Autodesk Inventor part; units mm, degrees
ref_plane "YZ Plane" through (0, 0, 0) normal (1, 0, 0) x (0, 1, 0)
ref_plane "XZ Plane" through (0, 0, 0) normal (0, 1, 0) x (-1, 0, 0)
ref_plane "XY Plane" through (0, 0, 0) normal (0, 0, 1) x (1, 0, 0)
sketch "スケッチ2" plane through (0, 0, 0) normal (0, 0, 1) x (1, 0, 0)
  line L0 (0, 0) -> (20, 0)
  line L1 (20, 0) -> (20, 80)
  line L2 (20, 80) -> (0, 80)
  line L3 (0, 80) -> (0, 0)
  line L4 (10, 80) -> (10, 0) construction
  circle A0 centre (10, 70) radius 2.75
  circle A1 centre (10, 10) radius 2.75
  dimension "d4" = 20
  dimension "d5" = 80
  dimension "d15" = 10
  dimension "d16" = 10
  dimension "d17" = 5.5
extrude "押し出し2" add sketch "スケッチ2" along normal blind 25
sketch "スケッチ4" plane through (0, 0, 25) normal (0, 0, 1) x (1, 0, 0)
  line L0 (0, 0) -> (20, 0) construction
  line L1 (10, 0) -> (10, 80) construction
  line L2 (20, 80) -> (0, 80) construction
  line L3 (0, 80) -> (0, 0) construction
  line L4 (0, 40) -> (20, 40) construction
  line L5 (20, 0) -> (20, 80) construction
  line L6 (13, 25) -> (7, 25)
  line L7 (7, 25) -> (7, 55)
  line L8 (7, 55) -> (13, 55)
  line L9 (13, 55) -> (13, 25)
  line L10 (13, 25) -> (7, 55) construction
  line L11 (7, 25) -> (13, 55) construction
  point P0 (10, 40)
  dimension "d18" = 6
  dimension "d19" = 30
extrude "押し出し4" add sketch "スケッチ4" along normal blind 2
fillet "フィレット1" radius 1 8 edges at (13, 25, 26) (13, 55, 26) (7, 55, 26) (7, 25, 26) (0, 0, 12.5) (20, 0, 12.5) (20, 80, 12.5) (0, 80, 12.5)
properties part number "モータースペーサ"
Could you check a few things on this model? Use its own coordinates, in mm. A direction names the side the tool comes from. Round coordinates to 2 decimals unless told otherwise and drop trailing zeros. Order: outer loops, then holes, each group sorted by start corner. A loop starts at its lowest first (then second) coordinate and runs counter-clockwise, first axis right, second up. Notation, with made-up numbers: M 47.25,-33 L 64.25,-33 A9 cw 64.25,-29 Z; hole C 62.5,-23.5 d6. An arc over 180 degrees is marked long. One line per item, written item: value.
(1) Which directions (+Z, -Z, +X, -X, +Y, -Y) give clear straight access to the entire face, cutting with the end or side of a thin tool? Please do faces 1 (the flat face through (10, 55, 26)), 2 (the flat face through (7, 40, 26)), 3 (the flat face through (10, 40, 27)), 4 (the flat face through (0, 41, 12)), 5 (the flat face through (14, 41, 25)).
Ans:
face 1: +Z, +X, -X, +Y
face 2: +Z, -X, +Y, -Y
face 3: +Z, +X, -X, +Y, -Y
face 4: +Z, -Z, -X, +Y, -Y
face 5: +Z
(2) Imagine slicing it at D-D (y = 33). Write out the boundary of the cut face in (x, z), and give its area (3 significant figures).
Ans:
outline: M 0,0 L 20,0 L 20,25 L 13,25 L 13,27 L 7,27 L 7,25 L 0,25 Z
area: 512 mm^2
(3) If we mould it in two halves opening along X, with no side actions, what happens to faces 6 (the flat face through (10, 25, 26)), 7 (the cylindrical face through (9.642, 67.273, 12.325)), 8 (the flat face through (13, 40, 26))? For each: released by +X, released by -X, zero draft, split by the parting line, or undercut.
Ans:
face 6: zero draft
face 7: undercut
face 8: released by +X
(4) Imagine slicing it at B-B (z = 17.5). Write out the boundary of the cut face in (x, y).
Ans:
outline: M 0,1 A1 ccw 1,0 L 19,0 A1 ccw 20,1 L 20,79 A1 ccw 19,80 L 1,80 A1 ccw 0,79 Z; hole C 10,10 d5.5; hole C 10,70 d5.5
(5) Imagine slicing it at C-C (y = 70). Write out the boundary of the cut face in (x, z).
Ans:
outline: M 0,0 L 7.25,0 L 7.25,25 L 0,25 Z; M 12.75,0 L 20,0 L 20,25 L 12.75,25 Z
(6) I need wall thicknesses on line 1 along Y through (x, z) = (10, 7.5); line 2 along Y through (x, z) = (8.5, 20.75); line 3 along Z through (x, y) = (2, 23.5). Which ranges of each line are inside material? Lowest first, please. Write a range as from..to.
Ans:
line 1: y = 0..7.25, 12.75..67.25, 72.75..80
line 2: y = 0..7.7, 12.3..67.7, 72.3..80
line 3: z = 0..25
(7) I'm going to push flat-ended pins straight in: P1, Ø0.6, axis at y = 46, z = 25.5, coming from the +X side; P2, Ø3.5, axis at x = 10, y = 10, coming from the -Z side; P3, Ø0.6, axis at y = 34.5, z = 26, coming from the -X side; P4, Ø0.6, axis at x = 9.5, z = 26.5, coming from the +Y side. Where does each tip first touch, or does it pass through?
Ans:
P1: stops at x = 13
P2: passes through
P3: stops at x = 7
P4: stops at y = 55
(8) Imagine slicing it at A-A (x = 10). Write out the boundary of the cut face in (y, z).
Ans:
outline: M 0,0 L 7.25,0 L 7.25,25 L 0,25 Z; M 12.75,0 L 67.25,0 L 67.25,25 L 55,25 L 55,27 L 25,27 L 25,25 L 12.75,25 Z; M 72.75,0 L 80,0 L 80,25 L 72.75,25 Z
